Input: part model. Units: mm. Frame: model coordinates. A direction names the side the tool comes from. Round coordinates to 2 decimals unless told otherwise and drop trailing zeros. Loops run counter-clockwise (first coordinate to the right, second up) from the corner with the lowest first, then second, coordinate; pieces in that order, holes last. Notation, with made-up numbers: M -25.75,48 L 26.25,48 A25 ccw 26.25,62 Z; hole C 52.25,-23 d10. An arc over 180 degrees is marked long. Return JSON: item names as keys, results as strings. Group by question number.
1) Section B-B (z = -1.5). Output: boundary loops of the cut face in (x, y), plus the area to 3 significant figures.
2) Section A-A (y = -16.5). Output: boundary loops of the cut face in (x, z), plus the area to 3 significant figures.
3) Section D-D (z = 13.5). Output: boundary loops of the cut face in (x, y), plus the area to 3 significant figures.
4) Material intervals for line 1 (Y direction, x = 0, z = -3.5); line 2 (Z direction, x = 15.5, y = 65.5); line 3 (Z direction, x = -1.5, y = 2), sorted ascending. Write a range as from..to.
5) Access query for faces 4 (the face through (-2.17, -37.74, 12.68)), 5 (the face through (0, 0, 1.5)), 6 (the face through (0, 18, -7.5)). Directions: +Z, -Z, +X, -X, +Y, -Y. A direction counts if a zero-diameter tool reaches every point of the face in a straight line with its end or side. Return the directions, or none.
6) Contact query for flat-ended pins moving along their axis: P1, Ø9, axis at x = 4.5, y = -3, coming from the -Z side; P2, Ø18, axis at x = 0, y = 0, coming from the +Z side; P3, Ø2, axis at y = 56.5, z = 14, coming from the -X side. Output: stop coordinate, or through.
7) Mould query, pull axis Y, two halves, no side actions, for faces 1 (the face through (-1.06, -55.56, 19.87)), 2 (the face through (0, 48, 20)), 3 (the face through (0, 72.5, -1)). Classes: +Y half, -Y half, draft (parallel to the pull), parting line (faces both ways), or undercut.
8) Section C-C (x = 0). Output: boundary loops of the cut face in (y, z).
Autodesk Inventor part; units mm, degrees
ref_plane "YZ Plane" through (0, 0, 0) normal (1, 0, 0) x (0, 1, 0)
ref_plane "XZ Plane" through (0, 0, 0) normal (0, 1, 0) x (-1, 0, 0)
ref_plane "XY Plane" through (0, 0, 0) normal (0, 0, 1) x (1, 0, 0)
sketch "Sketch1" plane through (0, 0, 0) normal (0, 0, 1) x (1, 0, 0)
  line L0 (223.4483, -72.5) -> (-46.5517, -72.5)
  line L1 (-46.5517, -72.5) -> (-46.5517, 72.5)
  line L2 (-46.5517, 72.5) -> (223.4483, 72.5)
  line L3 (223.4483, 72.5) -> (223.4483, -72.5)
  line L4 (223.4483, -72.5) -> (-46.5517, 72.5) construction
  line L5 (-46.5517, -72.5) -> (223.4483, 72.5) construction
  circle A0 centre (0, 47.5) radius 10
  line L6 (18, -72.5) -> (-18, -72.5)
  line L7 (-18, -72.5) -> (-18, 72.5)
  line L8 (-18, 72.5) -> (18, 72.5)
  line L9 (18, 72.5) -> (18, -72.5)
  line L10 (18, -72.5) -> (-18, 72.5) construction
  line L11 (-18, -72.5) -> (18, 72.5) construction
  line L12 (-100.5517, 0) -> (277.4483, 0) construction
  line L13 (0, 101.5) -> (0, -101.5) construction
  circle A1 centre (0, -47.5) radius 10
  line L14 (0, -101.5) -> (0, 101.5) construction
  circle A2 centre (0, 0) radius 15
  point P0 (88.4483, 0)
  dimension "d0" = 145
  dimension "d1" = 270
  dimension "d2" = 20
  dimension "d3" = 25
  dimension "d4" = 36
  dimension "d5" = 30
extrude "Extrusion1" add sketch "Sketch1" along normal mid plane 15 contours L0 L7 L2 L9
extrude "Extrusion2" add sketch "Sketch1" against normal blind 7.5 contours A0 | A1
extrude "Extrusion3" add sketch "Sketch1" along normal blind 20 contours A0 | A1
sketch "Sketch2" plane through (0, 0, 7.5) normal (0, 0, 1) x (1, 0, 0)
  line L0 (18, 72.5) -> (-18, 72.5)
  line L1 (-18, 72.5) -> (-18, -72.5)
  line L2 (-18, -72.5) -> (18, -72.5)
  line L3 (18, -72.5) -> (18, 72.5)
  circle A0 centre (0, 0) radius 15
  circle A1 centre (0, -47.5) radius 10
  circle A2 centre (0, 47.5) radius 10
extrude "Extrusion4" add sketch "Sketch2" against normal blind 6 contours A0
chamfer "Chamfer1" distance 2 angle 45 13 edges at (0, -72.5, 7.5) (18, -72.5, 0) (0, -72.5, -7.5) (18, 0, -7.5) (18, 0, 7.5) (18, 72.5, 0) (0, 72.5, 7.5) (-18, 0, 7.5) (-10, 47.5, 20) (-10, -47.5, 20) (-18, 0, -7.5) (-18, -72.5, 0) (-18, 72.5, 0)
properties part number "hydraulic_mech" material "Steel, Mild"
Returned:
{
 "1": {"outline": "M -18,-70.5 L -16,-72.5 L 16,-72.5 L 18,-70.5 L 18,70.5 L 16,72.5 L -16,72.5 L -18,70.5 Z; hole C 0,0 d30", "area": "4,510 mm^2"},
 "2": {"outline": "M -18,-5.5 L -16,-7.5 L 16,-7.5 L 18,-5.5 L 18,5.5 L 16,7.5 L -16,7.5 L -18,5.5 Z", "area": "532 mm^2"},
 "3": {"outline": "C 0,-47.5 d20; C 0,47.5 d20", "area": "628 mm^2"},
 "4": {"line 1": "y = -72.5..-15, 15..72.5", "line 2": "z = -7.5..7.5", "line 3": "z = 1.5..7.5"},
 "5": {"face 4": "+Z", "face 5": "-Z", "face 6": "-Z, +X, -X, +Y, -Y"},
 "6": {"P1": "stops at z = 1.5", "P2": "stops at z = 7.5", "P3": "stops at x = -6"},
 "7": {"face 1": "undercut", "face 2": "draft", "face 3": "+Y half"},
 "8": {"outline": "M -72.5,-5.5 L -70.5,-7.5 L -15,-7.5 L -15,1.5 L 15,1.5 L 15,-7.5 L 72.5,-7.5 L 72.5,5.5 L 70.5,7.5 L 57.5,7.5 L 57.5,18 L 55.5,20 L 39.5,20 L 37.5,18 L 37.5,7.5 L -37.5,7.5 L -37.5,18 L -39.5,20 L -55.5,20 L -57.5,18 L -57.5,7.5 L -70.5,7.5 L -72.5,5.5 Z"}
}
